```python
from build123d import *


with BuildPart() as part:
    # Sketch1 → Revolve1 (revolve)
    with BuildSketch(Plane.XY):
        with BuildLine():
            Line((18.5, 7), (18.5, 8))
            Line((18.5, 8), (10.5, 8))
            Line((10.5, 8), (9, 12.121216129))
            Line((9, 12.121216129), (5, 12.121216129))
            Line((5, 12.121216129), (5, 147.5))
            Line((5, 147.5), (2, 147.5))
            Line((2, 147.5), (2, 149.5))
            Line((2, 149.5), (3, 149.5))
            Line((3, 149.5), (3, 155.5))
            Line((3, 155.5), (0, 155.5))
            Line((0, 155.5), (0, 1))
            add(Edge.make_bspline(
                [(0, 1), (18.5, 1), (18.5, 7)],
                knots=[4.71238898, 4.71238898, 4.71238898, 6.283185307, 6.283185307, 6.283185307], degree=2, weights=[1, 0.707106781, 1]))
        make_face()
    revolve(axis=Axis((0, 0, 0), (0, 1, 0)))


solid = part.part
```
Part model, mm, in its own coordinate system. A direction names the side the tool comes from. Round coordinates to 2 decimals unless told otherwise and drop trailing zeros. Write each loop counter-clockwise with the first axis right and the second up, starting at its lowest first coordinate (ties: lowest second). Pieces come first, ordered by that corner, then holes. Notation, with made-up numbers: (8.25, 22.5) -> (42.25, 22.5) arc R10 cw to (42.25, 32.5) -> close; hole circle Ø9 at (-13.5, 61). An arc over 180 degrees is marked (long way). Return JSON: item names as keys, results as strings. Group by question number.
Q1. Mould opens along Y. For faces 4 (the cylindrical face through (-3, 153, 0)), 5 (the flat face through (-1, 149.5, 2)), 6 (the conical face through (8.654, 11.921, -2.725)), 7 (the flat face through (2.2, 147.5, -0.1)) say: pulls with the +Y half, pulls with the -Y half, needs draft (parallel to the pull), parting line crosses it, or undercut.
Q2. Saw through at A-A on y = 146. Write the cut outline in (x, z), plus the area to 3 significant figures.
Q3. Probe L1, parallel to X at y = 17, z = -4; L2, parallel to X at y = 41, z = 0.5. List the from-to ranges inside material, lowest first. Write a range as [from, to].
Q4. Which spindle directions (+Z, -Z, +X, -X, +Y, -Y) get a long thin tool onto all of the face, cutting with end or side? Do faces 1 (the flat face through (0, 155.5, 0)), 2 (the cylindrical face through (0, 149, 2)), 3 (the cylindrical face through (-1.08, 80.76, 4.88)). Say none if no direction does.
Q5. Pin check, flat tips, straight feed: pin 1 (3 mm diameter, centred on y = 104.5, z = 2.5, fed in from -X); pin 2 (2 mm diameter, centred on x = 3, y = 94, fed in from -Z); pin 3 (3 mm diameter, centred on y = 28, z = -5.5, fed in from -X); pin 4 (10 mm diameter, centred on y = 120, z = 11.5, fed in from +X). Stop position of each tip, or through.
Answer:
{
 "1": {"face 4": "needs draft", "face 5": "undercut", "face 6": "pulls with the +Y half", "face 7": "undercut"},
 "2": {"outline": "circle Ø10 at (0, 0)", "area": "78.5 mm2"},
 "3": {"L1": "[-3, 3]", "L2": "[-4.97, 4.97]"},
 "4": {"face 1": "+Z, -Z, +X, -X, +Y", "face 2": "none", "face 3": "+Y"},
 "5": {"pin 1": "x = -4.9", "pin 2": "z = -4.58", "pin 3": "x = -3", "pin 4": "through"}
}
